from build123d import *

# Parameters (mm, degrees)
SKETCH1_W           = 50.8
SKETCH1_H           = 50.8
SKETCH1_W_2         = 47.625
SKETCH1_H_2         = 47.625
BOSS_EXTRUDE1_DEPTH = 101.6
SKETCH2_R           = 2.54
CUT_EXTRUDE2_DEPTH  = 609.6
SKETCH3_R           = 2.54
CUT_EXTRUDE3_DEPTH  = 76.2


with BuildPart() as part:
    # Sketch1 → Boss-Extrude1 (new body)
    with BuildSketch(Plane(origin=(0, 0, 0), x_dir=(0, 0, -1), z_dir=(1, 0, 0))):
        Rectangle(SKETCH1_W, SKETCH1_H)
        Rectangle(SKETCH1_W_2, SKETCH1_H_2, mode=Mode.SUBTRACT)
    extrude(amount=BOSS_EXTRUDE1_DEPTH)

    # Sketch2 → Cut-Extrude2 (cut)
    with BuildSketch(Plane.XY.offset(25.4)):
        with Locations((12.7, 12.7)):
            Circle(SKETCH2_R)
        with Locations((12.7, 0)):
            Circle(SKETCH2_R)
        with Locations((12.7, -12.7)):
            Circle(SKETCH2_R)
        with Locations((25.4, 12.7)):
            Circle(SKETCH2_R)
        with Locations((25.4, 0)):
            Circle(SKETCH2_R)
        with Locations((25.4, -12.7)):
            Circle(SKETCH2_R)
        with Locations((38.1, 12.7)):
            Circle(SKETCH2_R)
        with Locations((38.1, 0)):
            Circle(SKETCH2_R)
        with Locations((38.1, -12.7)):
            Circle(SKETCH2_R)
        with Locations((50.8, 12.7)):
            Circle(SKETCH2_R)
        with Locations((50.8, 0)):
            Circle(SKETCH2_R)
        with Locations((50.8, -12.7)):
            Circle(SKETCH2_R)
        with Locations((63.5, 12.7)):
            Circle(SKETCH2_R)
        with Locations((63.5, 0)):
            Circle(SKETCH2_R)
        with Locations((63.5, -12.7)):
            Circle(SKETCH2_R)
        with Locations((76.2, 12.7)):
            Circle(SKETCH2_R)
        with Locations((76.2, 0)):
            Circle(SKETCH2_R)
        with Locations((76.2, -12.7)):
            Circle(SKETCH2_R)
        with Locations((88.9, 12.7)):
            Circle(SKETCH2_R)
        with Locations((88.9, 0)):
            Circle(SKETCH2_R)
        with Locations((88.9, -12.7)):
            Circle(SKETCH2_R)
    extrude(amount=-CUT_EXTRUDE2_DEPTH, mode=Mode.SUBTRACT)

    # Sketch3 → Cut-Extrude3 (cut)
    with BuildSketch(Plane.XZ.offset(25.4)):
        with Locations(Location((11.466852122, 12.7, 0), (0, 0, 270))):
            Circle(SKETCH3_R)
        with Locations(Location((11.466852122, 0, 0), (0, 0, 270))):
            Circle(SKETCH3_R)
        with Locations(Location((11.471230502, -12.699999245, 0), (0, 0, 270))):
            Circle(SKETCH3_R)
        with Locations(Location((24.166852122, 12.699999245, 0), (0, 0, 270))):
            Circle(SKETCH3_R)
        with Locations(Location((24.166852122, -7.55e-07, 0), (0, 0, 270))):
            Circle(SKETCH3_R)
        with Locations(Location((24.171230502, -12.7, 0), (0, 0, 270))):
            Circle(SKETCH3_R)
        with Locations(Location((36.866852122, 12.699999245, 0), (0, 0, 270))):
            Circle(SKETCH3_R)
        with Locations(Location((36.871230502, 0, 0), (0, 0, 270))):
            Circle(SKETCH3_R)
        with Locations(Location((36.871230502, -12.7, 0), (0, 0, 270))):
            Circle(SKETCH3_R)
        with Locations(Location((49.566852122, 12.699999245, 0), (0, 0, 270))):
            Circle(SKETCH3_R)
        with Locations(Location((49.571230502, 0, 0), (0, 0, 270))):
            Circle(SKETCH3_R)
        with Locations(Location((49.571230502, -12.7, 0), (0, 0, 270))):
            Circle(SKETCH3_R)
        with Locations(Location((62.266852122, 12.699999245, 0), (0, 0, 270))):
            Circle(SKETCH3_R)
        with Locations(Location((62.271230502, 0, 0), (0, 0, 270))):
            Circle(SKETCH3_R)
        with Locations(Location((62.271230502, -12.7, 0), (0, 0, 270))):
            Circle(SKETCH3_R)
        with Locations(Location((74.966852122, 12.699999245, 0), (0, 0, 270))):
            Circle(SKETCH3_R)
        with Locations(Location((74.971230502, 0, 0), (0, 0, 270))):
            Circle(SKETCH3_R)
        with Locations(Location((74.971230502, -12.7, 0), (0, 0, 270))):
            Circle(SKETCH3_R)
        with Locations(Location((87.671230502, 12.7, 0), (0, 0, 270))):
            Circle(SKETCH3_R)
        with Locations(Location((87.671230502, 0, 0), (0, 0, 270))):
            Circle(SKETCH3_R)
        with Locations(Location((87.671230502, -12.7, 0), (0, 0, 270))):
            Circle(SKETCH3_R)
    extrude(amount=-CUT_EXTRUDE3_DEPTH, mode=Mode.SUBTRACT)


solid = part.part
Design review of the part built by this model. Coordinates are the model's own, in mm. Round coordinates to 2 decimals unless told otherwise and drop trailing zeros. Write each loop counter-clockwise with the first axis right and the second up, starting at its lowest first coordinate (ties: lowest second). Pieces come first, ordered by that corner, then holes. Notation, with made-up numbers: (-12, 9.5) -> (18, 9.5) arc R16 cw to (18, 29.5) -> close; hole circle Ø5 at (18.5, -23). An arc over 180 degrees is marked (long way). One line per item, written item: value. Start each with the question number.
Q1. Add section D-D (z = -12.7). State how many separate pieces and enclosed holes the cut face has, then the cut area to 3 significant figures.
Q2. Add section C-C (x = 30). Give the boundary of the cut face in (y, z), then the cut area to 4 significant figures.
Q3. To check wall thickness, follow probe 1 along Y at (x, z) = (38.1, 24.2); probe 2 along Z at (x, y) = (24, 21.5). State the ranges of each line that lie inside material, in increasing order.
Q4. Add section A-A (z = -18). Give the boundary of the cut face in (x, y), then the cut area to 3 significant figures.
Response:
1. separate pieces: 16
1. enclosed holes: 0
1. area: 210 mm^2
2. outline: (-25.4, -25.4) -> (25.4, -25.4) -> (25.4, 25.4) -> (-25.4, 25.4) -> close; hole (-23.81, -23.81) -> (23.81, -23.81) -> (23.81, 23.81) -> (-23.81, 23.81) -> close
2. area: 312.5 mm^2
3. probe 1: y = -25.4 to -15.24, -10.16 to -2.54, 2.54 to 10.16, 15.24 to 25.4
3. probe 2: z = -25.4 to -23.81, 23.81 to 25.4
4. outline: (0, -25.4) -> (101.6, -25.4) -> (101.6, -23.81) -> (0, -23.81) -> close; (0, 23.81) -> (101.6, 23.81) -> (101.6, 25.4) -> (0, 25.4) -> close
4. area: 323 mm^2
